```python
from build123d import *

# Parameters (mm, degrees)
SALIENTE_EXTRUIR1_DEPTH = 60
CROQUIS2_R              = 1.6
CORTAR_EXTRUIR1_DEPTH   = 20
CORTAR_EXTRUIR2_START   = -10
CORTAR_EXTRUIR2_DEPTH   = 3
CROQUIS4_R              = 4.1
CORTAR_EXTRUIR3_DEPTH   = 64.639610307
CORTAR_EXTRUIR4_START   = -10
CROQUIS6_R              = 1.6
CORTAR_EXTRUIR4_DEPTH   = 10
CORTAR_EXTRUIR5_START   = -5
CORTAR_EXTRUIR5_DEPTH   = 30


with BuildPart() as part:
    # Croquis1 → Saliente-Extruir1 (new body)
    with BuildSketch(Plane.XY):
        Polygon((15, -6.213203436), (15, 6.213203436), (6.213203436, 15), (-6.213203436, 15), (-15, 6.213203436), (-15, -6.213203436), (-6.213203436, -15), (6.213203436, -15), align=None)
    extrude(amount=SALIENTE_EXTRUIR1_DEPTH)

    # Croquis2 → Cortar-Extruir1 (cut)
    with BuildSketch(Plane(origin=(0, 0, 0), x_dir=(-1, 0, 0), z_dir=(0, 0, -1))):
        with Locations((0, 11)):
            Circle(CROQUIS2_R)
        with Locations((7.778174593, 7.778174593)):
            Circle(CROQUIS2_R)
        with Locations((11, 0)):
            Circle(CROQUIS2_R)
        with Locations((7.778174593, -7.778174593)):
            Circle(CROQUIS2_R)
        with Locations((0, -11)):
            Circle(CROQUIS2_R)
        with Locations((-7.778174593, -7.778174593)):
            Circle(CROQUIS2_R)
        with Locations((-11, 0)):
            Circle(CROQUIS2_R)
        with Locations((-7.778174593, 7.778174593)):
            Circle(CROQUIS2_R)
    extrude(amount=-CORTAR_EXTRUIR1_DEPTH, mode=Mode.SUBTRACT)

    # Croquis3 → Cortar-Extruir2 (cut)
    with BuildSketch(Plane(origin=(0, 0, 0), x_dir=(-1, 0, 0), z_dir=(0, 0, -1)).offset(CORTAR_EXTRUIR2_START)):
        Polygon((-2.75, 12.58771324), (-2.75, 18.463203436), (2.75, 23.963203436), (2.75, 12.58771324), (2.75, 9.41228676), (0, 7.824573519), (-2.75, 9.41228676), align=None)
        Polygon((6.956313744, 10.84540104), (11.110912703, 15), (18.889087297, 15), (10.84540104, 6.956313744), (8.600035443, 4.710948146), (5.532808996, 5.532808996), (4.710948146, 8.600035443), align=None)
        Polygon((12.58771324, 2.75), (18.463203436, 2.75), (23.963203436, -2.75), (12.58771324, -2.75), (9.41228676, -2.75), (7.824573519, 0), (9.41228676, 2.75), align=None)
        Polygon((10.84540104, -6.956313744), (15, -11.110912703), (15, -18.889087297), (6.956313744, -10.84540104), (4.710948146, -8.600035443), (5.532808996, -5.532808996), (8.600035443, -4.710948146), align=None)
        Polygon((2.75, -12.58771324), (2.75, -18.463203436), (-2.75, -23.963203436), (-2.75, -12.58771324), (-2.75, -9.41228676), (0, -7.824573519), (2.75, -9.41228676), align=None)
        Polygon((-6.956313744, -10.84540104), (-11.110912703, -15), (-18.889087297, -15), (-10.84540104, -6.956313744), (-8.600035443, -4.710948146), (-5.532808995, -5.532808996), (-4.710948146, -8.600035443), align=None)
        Polygon((-12.58771324, -2.75), (-18.463203436, -2.75), (-23.963203436, 2.75), (-12.58771324, 2.75), (-9.41228676, 2.75), (-7.824573519, 0), (-9.41228676, -2.75), align=None)
        Polygon((-10.84540104, 6.956313744), (-15, 11.110912703), (-15, 18.889087297), (-6.956313744, 10.84540104), (-4.710948146, 8.600035443), (-5.532808996, 5.532808996), (-8.600035443, 4.710948146), align=None)
    extrude(amount=-CORTAR_EXTRUIR2_DEPTH, mode=Mode.SUBTRACT)

    # Croquis4 → Cortar-Extruir3 (cut, through all)
    with BuildSketch(Plane(origin=(0, 0, 0), x_dir=(-1, 0, 0), z_dir=(0, 0, -1))):
        Circle(CROQUIS4_R)
    extrude(amount=-CORTAR_EXTRUIR3_DEPTH, mode=Mode.SUBTRACT)

    # Croquis6 → Cortar-Extruir4 (cut)
    with BuildSketch(Plane.XY.offset(60).offset(CORTAR_EXTRUIR4_START)):
        with Locations(Location((0, 11, 0), (0, 0, 180))):
            Circle(CROQUIS6_R)
        with Locations(Location((7.778174593, 7.778174593, 0), (0, 0, 180))):
            Circle(CROQUIS6_R)
        with Locations(Location((11, 0, 0), (0, 0, 180))):
            Circle(CROQUIS6_R)
        with Locations(Location((7.778174593, -7.778174593, 0), (0, 0, 180))):
            Circle(CROQUIS6_R)
        with Locations(Location((0, -11, 0), (0, 0, 180))):
            Circle(CROQUIS6_R)
        with Locations(Location((-7.778174593, -7.778174593, 0), (0, 0, 180))):
            Circle(CROQUIS6_R)
        with Locations(Location((-11, 0, 0), (0, 0, 180))):
            Circle(CROQUIS6_R)
        with Locations(Location((-7.778174593, 7.778174593, 0), (0, 0, 180))):
            Circle(CROQUIS6_R)
    extrude(amount=CORTAR_EXTRUIR4_DEPTH, mode=Mode.SUBTRACT)

    # Croquis7 → Cortar-Extruir5 (cut)
    with BuildSketch(Plane.XY.offset(60).offset(CORTAR_EXTRUIR5_START)):
        with BuildLine():
            Line((-3, 11), (-3, 15))
            Line((-3, 15), (3, 15))
            Line((3, 15), (3, 11))
            ThreePointArc((3, 11), (0, 8), (-3, 11))
        make_face()
        with BuildLine():
            Line((5.656854249, 9.899494937), (8.485281374, 12.727922061))
            Line((8.485281374, 12.727922061), (12.727922061, 8.485281374))
            Line((12.727922061, 8.485281374), (9.899494937, 5.656854249))
            ThreePointArc((9.899494937, 5.656854249), (5.656854249, 5.656854249), (5.656854249, 9.899494937))
        make_face()
        with BuildLine():
            Line((11, 3), (15, 3))
            Line((15, 3), (15, -3))
            Line((15, -3), (11, -3))
            ThreePointArc((11, -3), (8, 0), (11, 3))
        make_face()
        with BuildLine():
            Line((9.899494937, -5.656854249), (12.727922061, -8.485281374))
            Line((12.727922061, -8.485281374), (8.485281374, -12.727922061))
            Line((8.485281374, -12.727922061), (5.656854249, -9.899494937))
            ThreePointArc((5.656854249, -9.899494937), (5.656854249, -5.656854249), (9.899494937, -5.656854249))
        make_face()
        with BuildLine():
            Line((3, -11), (3, -15))
            Line((3, -15), (-3, -15))
            Line((-3, -15), (-3, -11))
            ThreePointArc((-3, -11), (0, -8), (3, -11))
        make_face()
        with BuildLine():
            Line((-5.656854249, -9.899494937), (-8.485281374, -12.727922061))
            Line((-8.485281374, -12.727922061), (-12.727922061, -8.485281374))
            Line((-12.727922061, -8.485281374), (-9.899494937, -5.656854249))
            ThreePointArc((-9.899494937, -5.656854249), (-5.656854249, -5.656854249), (-5.656854249, -9.899494937))
        make_face()
        with BuildLine():
            Line((-11, -3), (-15, -3))
            Line((-15, -3), (-15, 3))
            Line((-15, 3), (-11, 3))
            ThreePointArc((-11, 3), (-8, 0), (-11, -3))
        make_face()
        with BuildLine():
            Line((-9.899494937, 5.656854249), (-12.727922061, 8.485281374))
            Line((-12.727922061, 8.485281374), (-8.485281374, 12.727922061))
            Line((-8.485281374, 12.727922061), (-5.656854249, 9.899494937))
            ThreePointArc((-5.656854249, 9.899494937), (-5.656854249, 5.656854249), (-9.899494937, 5.656854249))
        make_face()
    extrude(amount=-CORTAR_EXTRUIR5_DEPTH, mode=Mode.SUBTRACT)


solid = part.part
```
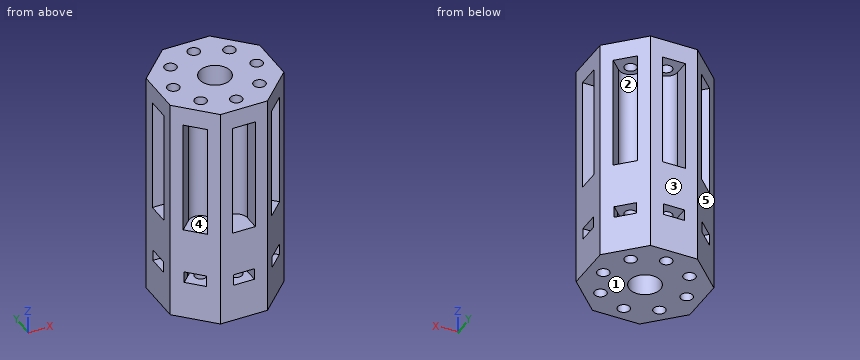
For this review, take the finished solid that the model builds, in its own axes (mm). Face numbers are marked on the shaded views. A direction names the side the tool comes from. Give positions to 0.01 mm unless a question says otherwise; leave off trailing zeros. Answer as a JSON object with one key per item and string values. Group by question number.
Item 1: Draft analysis for pull direction Y (two halves, no side actions). For the marked faces 1, 2 and 3, state which applies: +Y half, -Y half, draft (parallel to the pull), parting line (faces both ways), or undercut.
Item 2: For probe 1 along Z at (x, y) = (-8.5, -11.75); probe 2 along Z at (x, y) = (7.5, -11.5); probe 3 along Y at (x, z) = (-0.25, 26.5), list the stretches that pass through material, from the lowest coordinate up. Write a range as [from, to].
Item 3: Tool access review of the marked faces 4 and 5: name each direction out of +Z, -Z, +X, -X, +Y, -Y from which nothing blocks a thin tool from reaching the whole face with its end or side.
Item 4: For pin 1 Ø4 at (x, y) = (7.78, 7.78) entering from +Z; pin 2 Ø1.9 at (x, y) = (-7.78, 7.78) entering from -Z; pin 3 Ø8 at (y, z) = (-11.5, 44.5) entering from +X; pin 4 Ø5 at (x, z) = (-9, 36.5) entering from -Y, all flat-tipped, find the tip position at first contact; note any pin that passes through.
Item 5: Consider section A-A on z = 14.5. Count the separate pieces of the cut face and the enclosed holes in it, plus the area to 3 significant figures.
Check result:
{
 "1": {"face 1": "draft", "face 2": "undercut", "face 3": "+Y half"},
 "2": {"probe 1": "z = [0, 10], [13, 25], [55, 60]", "probe 2": "z = [0, 25], [55, 60]", "probe 3": "y = [-8.01, -4.09], [4.09, 8.01]"},
 "3": {"face 4": "none", "face 5": "+Z, -Z, -X, +Y"},
 "4": {"pin 1": "stops at z = 60", "pin 2": "stops at z = 20", "pin 3": "stops at x = 13.71", "pin 4": "stops at y = -14.71"},
 "5": {"separate pieces": "1", "enclosed holes": "9", "area": "628 mm^2"}
}
